Geometry check sheet. Reference: the model listing, model coordinates, mm. Round coordinates to 2 decimals unless told otherwise and drop trailing zeros. Write each loop counter-clockwise with the first axis right and the second up, starting at its lowest first coordinate (ties: lowest second). Pieces come first, ordered by that corner, then holes. Notation, with made-up numbers: (-27, -6) -> (-1, -6) arc R19 cw to (-1, 10) -> close; hole circle Ø9 at (53, 28). An arc over 180 degrees is marked (long way). One line per question, with ' | ' between items.
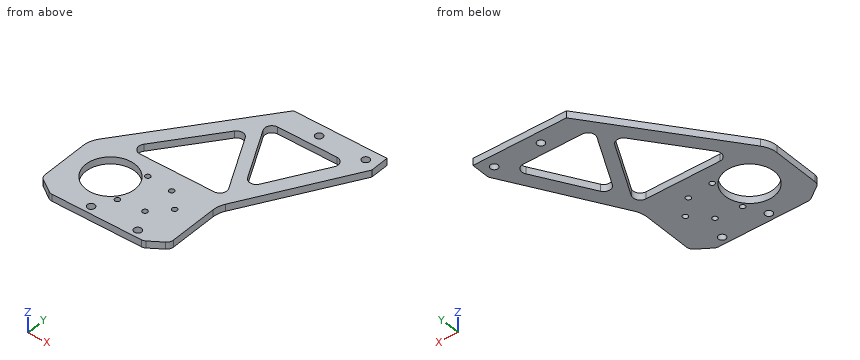
```python
from build123d import *

# Parameters (mm, degrees)
EXTRUDE_3_DEPTH     = 3
SKETCH_6_R          = 1.6
SKETCH_6_R_2        = 1.1
SKETCH_6_R_3        = 10.5
CUT_EXTRUDE_1_DEPTH = 106.547382725
CUT_EXTRUDE_2_DEPTH = 10
FILLET_1_R          = 10
FILLET_2_R          = 3


with BuildPart() as part:
    # 草图5 → 凸台-拉伸3 (new body)
    with BuildSketch(Plane.XY):
        Polygon((-20, 0), (20, 0), (20, -8), (-7.5, -55), (-7.5, -80), (-15, -85), (-55, -85), (-62.5, -80), (-62.5, -55), align=None)
    extrude(amount=EXTRUDE_3_DEPTH)

    # 草图6 → 切除-拉伸1 (cut, through all)
    with BuildSketch(Plane.XY.offset(3)):
        with Locations((-5, -5)):
            Circle(SKETCH_6_R)
        with Locations((15, -5)):
            Circle(SKETCH_6_R)
        with Locations((-40, -81.8)):
            Circle(SKETCH_6_R)
        with Locations((-20, -81.8)):
            Circle(SKETCH_6_R)
        with Locations((-17.5, -65.5)):
            Circle(SKETCH_6_R_2)
        with Locations((-24.5, -58.5)):
            Circle(SKETCH_6_R_2)
        with Locations((-35.5, -57.5)):
            Circle(SKETCH_6_R_2)
        with Locations(Location((-35.5, -73.5, 0), (0, 0, 180))):
            Circle(SKETCH_6_R_2)
        with Locations(Location((-24.5, -72.5, 0), (0, 0, 180))):
            Circle(SKETCH_6_R_2)
        with Locations((-45, -65.5)):
            Circle(SKETCH_6_R_3)
    extrude(amount=-CUT_EXTRUDE_1_DEPTH, mode=Mode.SUBTRACT)

    # 草图7 → 切除-拉伸2 (cut)
    with BuildSketch(Plane.XY.offset(3)):
        with BuildLine():
            Line((-28.443219333, -20.739299448), (-47.318132371, -45.165657497))
            ThreePointArc((-47.318132371, -45.165657497), (-47.637140852, -48.322303386), (-44.944277366, -50))
            Line((-44.944277366, -50), (-13.246531534, -50))
            ThreePointArc((-13.246531534, -50), (-10.67911571, -48.551894323), (-10.590292839, -45.605583994))
            Line((-10.590292839, -45.605583994), (-23.413125634, -21.179225945))
            ThreePointArc((-23.413125634, -21.179225945), (-25.807985355, -19.585050137), (-28.443219333, -20.739299448))
        make_face()
        with BuildLine():
            Line((-4.108825767, -37.323278412), (9.236421762, -14.515037181))
            ThreePointArc((9.236421762, -14.515037181), (9.249498939, -11.507537529), (6.647085488, -10))
            Line((6.647085488, -10), (-18.671550094, -10))
            ThreePointArc((-18.671550094, -10), (-21.238965917, -11.448105677), (-21.327788788, -14.394416006))
            Line((-21.327788788, -14.394416006), (-9.354400735, -37.202657237))
            ThreePointArc((-9.354400735, -37.202657237), (-6.76712834, -38.8074484), (-4.108825767, -37.323278412))
        make_face()
    extrude(amount=-CUT_EXTRUDE_2_DEPTH, mode=Mode.SUBTRACT)

    # 圆角1
    fillet_1_edges = [part.edges().sort_by_distance(p)[0] for p in [
        (-62.5, -55, 1.5),
        (-7.5, -55, 1.5),
    ]]
    fillet(fillet_1_edges, radius=FILLET_1_R)

    # 圆角2
    fillet_2_edges = [part.edges().sort_by_distance(p)[0] for p in [
        (-62.5, -80, 1.5),
        (-7.5, -80, 1.5),
        (-15, -85, 1.5),
        (-55, -85, 1.5),
    ]]
    fillet(fillet_2_edges, radius=FILLET_2_R)


solid = part.part
```
(1) Sectioned sample at B-B on x = 0.5. Record the cut outline in (y, z).
Resolved:
outline: (-41.33, 0) -> (-29.45, 0) -> (-29.45, 3) -> (-41.33, 3) -> close; (-10, 0) -> (0, 0) -> (0, 3) -> (-10, 3) -> close
(2) Material ranges on line 1 (Y direction, x = -35.5, z = 2.2); line 2 (X direction, y = -72.5, z = 2.3); line 3 (Y direction, x = -5, z = 2.35), recorded low to high.
Resolved:
line 1: y = -85 to -74.6, -72.4 to -69.97, -61.03 to -58.6, -56.4 to -50, -29.87 to -20.06 | line 2: x = -62.5 to -52.83, -37.17 to -35.96, -35.04 to -25.6, -23.4 to -7.5 | line 3: y = -50.73 to -38.28, -10 to -6.6, -3.4 to 0
(3) Go/stop test with flat-tipped pins: pin 1 (1.3 mm diameter, centred on x = -24.5, y = -72.5, fed in from -Z); pin 2 (1.5 mm diameter, centred on y = -63, z = 1, fed in from +X); pin 3 (1.5 mm diameter, centred on x = -30, z = 1.5, fed in from +Y); pin 4 (1.5 mm diameter, centred on x = -6, z = 1.5, fed in from -Y). Record where each tip stops, or that it passes through.
Resolved:
pin 1: passes through | pin 2: stops at x = -7.5 | pin 3: stops at y = -11.97 | pin 4: stops at y = -53.91
(4) Sectioned sample at C-C on y = -17. Record the cut outline in (x, z), then the cut area to 3 significant figures.
Resolved:
outline: (-33.14, 0) -> (-19.96, 0) -> (-19.96, 3) -> (-33.14, 3) -> close; (7.78, 0) -> (14.73, 0) -> (14.73, 3) -> (7.78, 3) -> close | area: 60.4 mm2
(5) Sectioned sample at A-A on y = -31. Record the cut outline in (x, z).
Resolved:
outline: (-43.95, 0) -> (-36.37, 0) -> (-36.37, 3) -> (-43.95, 3) -> close; (-18.26, 0) -> (-12.61, 0) -> (-12.61, 3) -> (-18.26, 3) -> close; (-0.41, 0) -> (6.54, 0) -> (6.54, 3) -> (-0.41, 3) -> close
(6) Sectioned sample at D-D on x = -39.5. Record the cut outline in (y, z), then the cut area to 3 significant figures.
Resolved:
outline: (-85, 0) -> (-83.32, 0) -> (-83.32, 3) -> (-85, 3) -> close; (-80.28, 0) -> (-74.44, 0) -> (-74.44, 3) -> (-80.28, 3) -> close; (-56.56, 0) -> (-50, 0) -> (-50, 3) -> (-56.56, 3) -> close; (-35.05, 0) -> (-25.24, 0) -> (-25.24, 3) -> (-35.05, 3) -> close | area: 71.7 mm2
